Geometry check sheet. Reference: drawing and pictorial views, mm from the part's lowest x, y, z. A direction names the side the tool comes from. Round coordinates to 2 decimals unless told otherwise and drop trailing zeros. Order: outer loops, then holes, each group sorted by start corner. A loop starts at its lowest first (then second) coordinate and runs counter-clockwise, first axis right, second up.
(1) Gauge pin test, flat ends, axial feed: P1, Ø1, axis at x = 23.5, z = 1.5, coming from the -Y side; P2, Ø0.6, axis at x = 3, z = 1.5, coming from the -Y side; P3, Ø0.6, axis at x = 3.5, z = 0.5, coming from the +Y side; P4, Ø3, axis at x = 5, y = 7, coming from the -Z side. Record the tip position at first contact, or that the pin passes through.
(2) Cross-section at C-C on y = 5.5. Count the separate pieces of the cut face and the enclosed holes in it, and give its area (3 significant figures).
(3) Thickness scan on L1, parallel to Y at x = 2.75, z = 0.25; L2, parallel to X at y = 18.25, z = 0.35; L3, parallel to X at y = 19.25, z = 1. Record the ranges inside material, lowest first.
(4) Draft check along Y on the marked faces 1, 2, 3 and 4. Enter one of: pulls with the +Y half, pulls with the -Y half, needs draft (parallel to the pull), parting line crosses it, or undercut.
(5) Cross-section at B-B on z = 1. Enter the section's corners in (x, y), and give its area (3 significant figures).
(6) Cross-section at A-A on x = 12.5. Enter the section's corners in (y, z), and give its area (3 significant figures).
(7) Set-up check for the marked faces 5 and 6: record each of +Z, -Z, +X, -X, +Y, -Y from which the full face is reachable in a straight line by a thin tool's end or side.
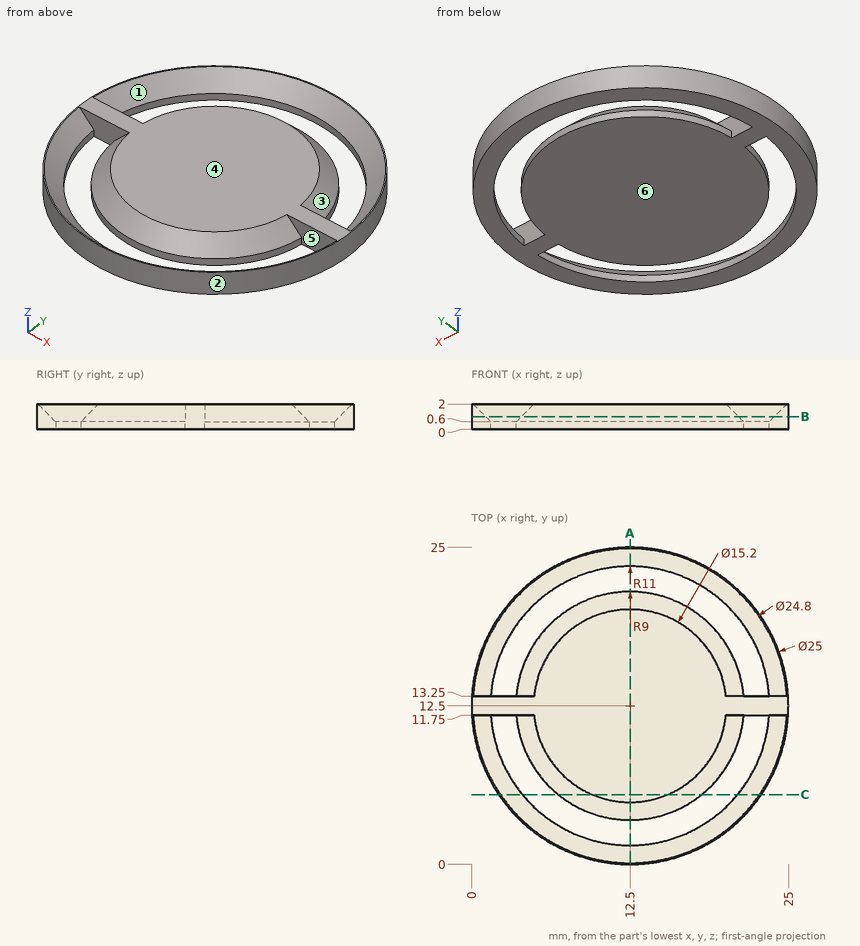
Found:
1. P1: stops at y = 5.72
1. P2: stops at y = 4.04
1. P3: stops at y = 21.48
1. P4: stops at z = 0
2. separate pieces: 3
2. enclosed holes: 0
2. area: 24.1 mm2
3. L1: y = 4.68 to 7.41, 11.75 to 13.25, 17.59 to 20.32
3. L2: x = 1.4 to 3.12, 5.58 to 19.42, 21.88 to 23.6
3. L3: x = 1.98 to 3.31, 7.17 to 17.83, 21.69 to 23.02
4. face 1: undercut
4. face 2: parting line crosses it
4. face 3: undercut
4. face 4: needs draft
5. outline: circle Ø25 at (12.5, 12.5); hole (1.12, 11.75) arc R11.4 ccw to (23.88, 11.75) - (21.07, 11.75) arc R8.6 cw to (3.93, 11.75) - close; hole (1.12, 13.25) - (3.93, 13.25) arc R8.6 cw to (21.07, 13.25) - (23.88, 13.25) arc R11.4 ccw to start
5. area: 323 mm2
6. outline: (0, 0) - (1.5, 0) - (1.5, 0.6) - (0.1, 2) - (0, 2) - close; (3.5, 0) - (21.5, 0) - (21.5, 0.6) - (20.1, 2) - (4.9, 2) - (3.5, 0.6) - close; (23.5, 0) - (25, 0) - (25, 2) - (24.9, 2) - (23.5, 0.6) - close
6. area: 38.1 mm2
7. face 5: +Z
7. face 6: -Z, +X, -X, +Y, -Y
